Model file for the job. Use its own axes, mm. A direction names the side the tool comes from. Coordinates: 2 decimals unless noted, no trailing zeros. Write each loop counter-clockwise with the first axis right and the second up, starting at its lowest first coordinate (ties: lowest second). Pieces come first, ordered by that corner, then holes.
Q1. Band-saw the part on D-D, the plane x = 5. Write the cut outline in (y, z).
Q2. Band-saw the part on B-B, the plane z = 12.25. Write the cut outline in (x, y), plus the area to 3 significant figures.
Q3. Band-saw the part on C-C, the plane x = 30. Write the cut outline in (y, z).
Q4. Drill centre lines: probe 1 along Y at (x, z) = (5, 12.75); probe 2 along Y at (x, z) = (30, 6); probe 3 along Z at (x, y) = (19.5, 7.75). Where is each one in solid material? Low to high.
Q5. Pin check, flat tips, straight feed: P1, Ø12, axis at x = 16.5, y = 10, coming from the -Z side; P2, Ø3, axis at y = 13, z = -7, coming from the -X side; P3, Ø4, axis at x = 12.5, y = 8, coming from the -Z side; P4, Ø6, axis at x = 30, y = 10, coming from the -Z side. Stop position of each tip, or through.
Q6. Band-saw the part on A-A, the plane y = 15. Write the cut outline in (x, z), plus the area to 3 significant figures.
Q7. Pull direction X, two halves, no side cores. Call faces 1 (the cylindrical face through (6.386, 4.425, 9.126)), 2 (the flat face through (20, 10, 18)), 3 (the flat face through (0, 10, 9)): released by +X, released by -X, zero draft, split by the parting line, or undercut.
Q8. Which spindle directions (+Z, -Z, +X, -X, +Y, -Y) get a long thin tool onto all of the face, cutting with end or side? Do faces 4 (the flat face through (20, 10, -5)), 5 (the flat face through (40, 10, 4)). Say none if no direction does.
from build123d import *

# Parameters (mm, degrees)
SKETCH1_W           = 40
SKETCH1_H           = 20
BOSS_EXTRUDE1_DEPTH = 18
SKETCH3_W           = 20
SKETCH3_H           = 20
BOSS_EXTRUDE2_DEPTH = 10
SKETCH2_R           = 3.25
SKETCH2_R_2         = 1.5
CUT_EXTRUDE1_DEPTH  = 65


with BuildPart() as part:
    # Sketch1 → Boss-Extrude1 (new body)
    with BuildSketch(Plane.XY):
        with Locations((20, 10)):
            Rectangle(SKETCH1_W, SKETCH1_H)
    extrude(amount=BOSS_EXTRUDE1_DEPTH)

    # Sketch3 → Boss-Extrude2 (add)
    with BuildSketch(Plane(origin=(0, 0, 0), x_dir=(-1, 0, 0), z_dir=(0, 0, -1))):
        with Locations((-30, 10)):
            Rectangle(SKETCH3_W, SKETCH3_H)
    extrude(amount=BOSS_EXTRUDE2_DEPTH)

    # Sketch2 → Cut-Extrude1 (cut)
    with BuildSketch(Plane.XY.offset(18)):
        with Locations((30, 10)):
            Circle(SKETCH2_R)
        with Locations((5, 15)):
            Circle(SKETCH2_R_2)
        with Locations((5, 5)):
            Circle(SKETCH2_R_2)
    extrude(amount=-CUT_EXTRUDE1_DEPTH, mode=Mode.SUBTRACT)


solid = part.part
Answer sheet:
1. outline: (0, 0) - (3.5, 0) - (3.5, 18) - (0, 18) - close; (6.5, 0) - (13.5, 0) - (13.5, 18) - (6.5, 18) - close; (16.5, 0) - (20, 0) - (20, 18) - (16.5, 18) - close
2. outline: (0, 0) - (40, 0) - (40, 20) - (0, 20) - close; hole circle Ø3 at (5, 5); hole circle Ø3 at (5, 15); hole circle Ø6.5 at (30, 10)
2. area: 753 mm2
3. outline: (0, -10) - (6.75, -10) - (6.75, 18) - (0, 18) - close; (13.25, -10) - (20, -10) - (20, 18) - (13.25, 18) - close
4. probe 1: y = 0 to 3.5, 6.5 to 13.5, 16.5 to 20
4. probe 2: y = 0 to 6.75, 13.25 to 20
4. probe 3: z = 0 to 18
5. P1: stops at z = -10
5. P2: stops at x = 20
5. P3: stops at z = 0
5. P4: passes through
6. outline: (0, 0) - (3.5, 0) - (3.5, 18) - (0, 18) - close; (6.5, 0) - (20, 0) - (20, -10) - (40, -10) - (40, 18) - (6.5, 18) - close
6. area: 866 mm2
7. face 1: undercut
7. face 2: zero draft
7. face 3: released by -X
8. face 4: -Z, -X, +Y, -Y
8. face 5: +Z, -Z, +X, +Y, -Y
